The figure shows three views and two pictorial views of one solid part (mm, origin at its lowest corner). Answer the questions. A direction names the side the tool comes from. Coordinates: 2 decimals unless noted, no trailing zeros. Write each loop counter-clockwise with the first axis right and the second up, starting at its lowest first coordinate (ties: lowest second). Pieces come first, ordered by that corner, then holes. Notation, with made-up numbers: (46, 20) - (59, 20) arc R13 ccw to (59, 38) - close; hole circle Ø1 at (25, -10). An arc over 180 degrees is marked (long way). Use a Markdown table: item, result. Add a question column.
(1) The part is cut by section B-B, the plane z = 8. Give the vertices of the cut face in (x, y).
(2) For a pull along X with two mould halves and no side action, classify the marked faces 3, 4 and 5 as released by +X, released by -X, zero draft, split by the parting line, or undercut.
(3) Given pin 1 Ø12.5 at (x, y) = (16, 13) entering from +Z; pin 2 Ø4 at (y, z) = (21, 12) entering from -X; pin 3 Ø2 at (x, y) = (17.5, 1.5) entering from +Z, each flat-ended and moving along its own axis, determine where each tip first touches the part or whether it passes through.
(4) Find the intervals of material crossed by line 1 (X direction, y = 18.75, z = 7.75); line 2 (Y direction, x = 6.5, z = 9.5); line 3 (Z direction, x = 9.5, y = 15.5), in increasing order. Write a range as from..to.
(5) A tool of negligible diameter and unlimited length cuts with its end or side. For the marked faces 1 and 2, from which of +Z, -Z, +X, -X, +Y, -Y can it reach the whole face along a straight path? Write none if from no direction.
(6) The part is cut by section D-D, the plane z = 10. Give the vertices of the cut face in (x, y), then the cut area to 3 significant figures.
(7) The part is cut by section A-A, the plane y = 17. Give the vertices of the cut face in (x, z).
(8) The part is cut by section C-C, the plane x = 8. Give the vertices of the cut face in (y, z).
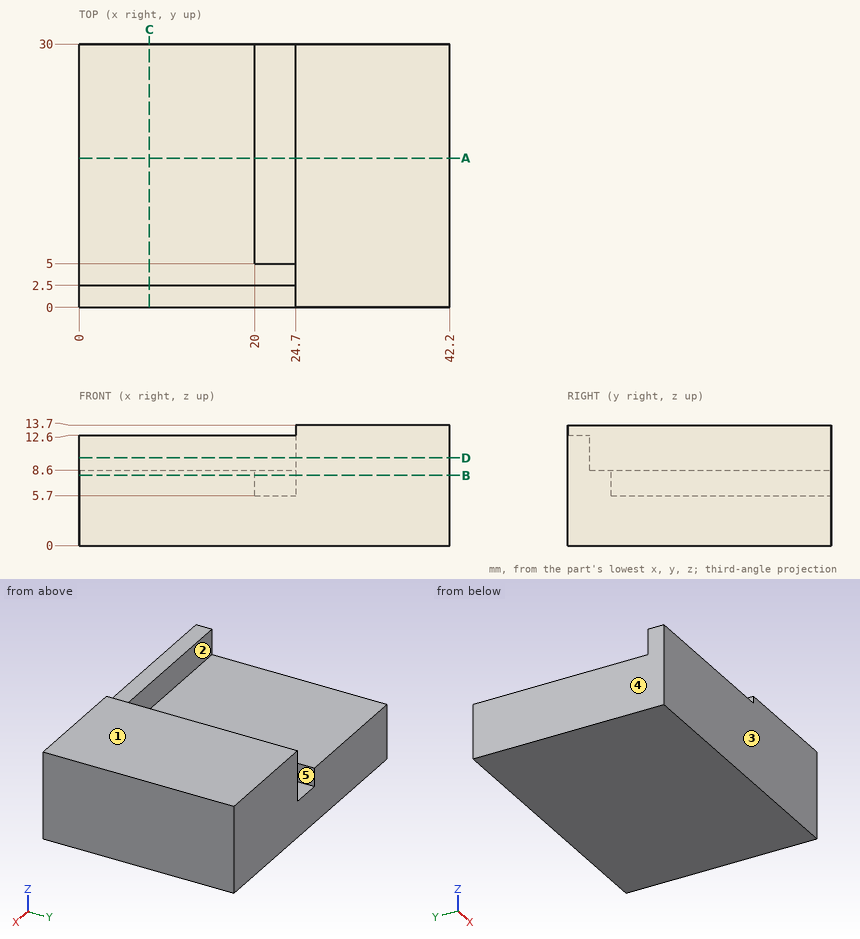
Model answer:
| question | item | result |
|---|---|---|
| 1 | outline | (0, 0) - (42.2, 0) - (42.2, 30) - (24.7, 30) - (24.7, 5) - (20, 5) - (20, 30) - (0, 30) - close |
| 2 | face 3 | zero draft |
| 2 | face 4 | released by -X |
| 2 | face 5 | undercut |
| 3 | pin 1 | z = 8.6 |
| 3 | pin 2 | x = 24.7 |
| 3 | pin 3 | z = 12.6 |
| 4 | line 1 | 0..20, 24.7..42.2 |
| 4 | line 2 | 0..2.5 |
| 4 | line 3 | 0..8.6 |
| 5 | face 1 | +Z, +X, -X, +Y, -Y |
| 5 | face 2 | +Z, -X, +Y |
| 6 | outline | (0, 0) - (42.2, 0) - (42.2, 30) - (24.7, 30) - (24.7, 2.5) - (0, 2.5) - close |
| 6 | area | 587 mm^2 |
| 7 | outline | (0, 0) - (42.2, 0) - (42.2, 13.7) - (24.7, 13.7) - (24.7, 5.7) - (20, 5.7) - (20, 8.6) - (0, 8.6) - close |
| 8 | outline | (0, 0) - (30, 0) - (30, 8.6) - (2.5, 8.6) - (2.5, 12.6) - (0, 12.6) - close |
